Read the model definition and answer for the solid it produces. Units are mm, in the model's axes. A direction names the side the tool comes from. Round coordinates to 2 decimals unless told otherwise and drop trailing zeros. Order: outer loops, then holes, each group sorted by start corner. A loop starts at its lowest first (then second) coordinate and runs counter-clockwise, first axis right, second up. Notation, with made-up numbers: (-35.75, 66) - (1.25, 66) arc R18 ccw to (1.25, 71) - close; hole circle Ø3 at (89, 79.25). An arc over 180 degrees is marked (long way). Answer as a JSON object with one key per item and string values. Group by question number.
Q1. Given pin 1 Ø1.5 at (x, z) = (-5, 4) entering from -Y; pin 2 Ø0.6 at (y, z) = (-1.5, 0.5) entering from -X; pin 3 Ø3 at (x, y) = (-7, -2.5) entering from +Z; pin 4 Ø2.5 at (x, z) = (11, 3.5) entering from -Y, each flat-ended and moving along its own axis, determine where each tip first touches the part or whether it passes through.
Q2. Consider line 1 (Z direction, x = -11, y = -11.2); line 2 (X direction, y = 5, z = 0.75); line 3 (Z direction, x = -8.75, y = 4.5). Determine where each line is inside the solid, lowest interval first.
Q3. A cutting plane is placed at A-A on z = 1.5. Determine the outline of the cut face in (x, y).
Q4. A cutting plane is placed at C-C on x = -10.5. Determine the outline of the cut face in (y, z), and give its area (3 significant figures).
Q5. A cutting plane is placed at D-D on z = 3.5. Count the separate pieces of the cut face and the enclosed holes in it, and give its area (3 significant figures).
Q6. The mould has two halves that part along Y. Classify faces 5 (the flat face through (-6, 10, 4)), 6 (the flat face through (9, -10, 4)), 7 (the cylindrical face through (9.5, -7.46, 3.57)): pulls with the +Y half, pulls with the -Y half, needs draft (parallel to the pull), parting line crosses it, or undercut.
Q7. A tool of negligible diameter and unlimited length cuts with its end or side. For faces 1 (the flat face through (10.5, 7.5, 1)), 2 (the flat face through (-7, -15, 4)), 3 (the cylindrical face through (7.056, -10.245, 3.465)), 4 (the flat face through (-10.5, 12.5, 1)), from which of +Z, -Z, +X, -X, +Y, -Y can it reach the whole face along a straight path? Write none if from no direction.
Q8. A cutting plane is placed at B-B on y = 12. Determine the outline of the cut face in (x, z), and give its area (3 significant figures).
```python
from build123d import *

# Parameters (mm, degrees)
F0_W          = 20
F0_H          = 1
F1_DEPTH      = 20
F1_DEPTH_BACK = 20
F3_DEPTH      = 40
F5_DEPTH      = 5
F7_R          = 1.5
F8_DEPTH      = 20.001
F8_DEPTH_BACK = 20.001
F9_R          = 5


# Not quite as in the source:
# - a pattern or mirror of a feature is missing from the dataset's text; its kind, count and spacing are read off the source's solid


with BuildPart() as f1:
    # F0 (on Front) → F1 (new body, two sides)
    with BuildSketch(Plane.XZ) as f1_sk:
        with Locations((0, -0.5)):
            Rectangle(F0_W, F0_H)
    extrude(amount=F1_DEPTH)
    extrude(f1_sk.sketch, amount=-F1_DEPTH_BACK)

    # F2 (on face) → F3 (join, through all)
    with BuildSketch(Plane(origin=(0, 20, 0), x_dir=(-1, 0, 0), z_dir=(0, 1, 0))):
        with BuildLine():
            Line((10, 1), (11, 1))
            ThreePointArc((11, 1), (13.5, 3.5), (11, 6))
            Line((11, 6), (0, 6))
            Line((0, 6), (-11, 6))
            ThreePointArc((-11, 6), (-13.5, 3.5), (-11, 1))
            Line((-11, 1), (-10, 1))
            Line((-10, 1), (-10, 0))
            Line((-10, 0), (0, 0))
            Line((0, 0), (10, 0))
            Line((10, 0), (10, 1))
        make_face()
    extrude(amount=-F3_DEPTH)

    # F4 (on face) → F5 (cut, through all)
    with BuildSketch(Plane.XY.offset(6)):
        Polygon((0, -15), (-13.5, -15), (-13.5, -20), (13.5, -20), (13.5, -10), (7, -10), align=None)
        Polygon((-13.5, 0), (-13.5, -10), (0, -10), (7, -5), (13.5, -5), (13.5, 0), align=None)
    f5 = extrude(amount=-F5_DEPTH, mode=Mode.SUBTRACT)

    # F5_copies: F5 across plane
    add(f5.mirror(Plane.ZX), mode=Mode.SUBTRACT)

    # F7 (on offset) → F8 (cut, two sides)
    with BuildSketch(Plane.XZ) as f8_sk:
        with Locations((11, 3.5)):
            Circle(F7_R)
        with Locations((-11, 3.5)):
            Circle(F7_R)
    extrude(amount=-F8_DEPTH, mode=Mode.SUBTRACT)
    extrude(f8_sk.sketch, amount=F8_DEPTH_BACK, mode=Mode.SUBTRACT)

    # F9
    f9_edges = [f1.edges().sort_by_distance(p)[0] for p in [
        (0, -15, 3.5),
        (0, -10, 3.5),
        (7, -5, 3.5),
        (7, -10, 3.5),
        (7, 10, 3.5),
        (0, 15, 3.5),
        (0, 10, 3.5),
        (7, 5, 3.5),
    ]]
    fillet(f9_edges, radius=F9_R)


solid = f1.part
```
Result set:
{
 "1": {"pin 1": "stops at y = -15", "pin 2": "stops at x = -10", "pin 3": "stops at z = 1", "pin 4": "passes through"},
 "2": {"line 1": "z = 1 to 2, 5 to 6", "line 2": "x = -10 to 10", "line 3": "z = -1 to 1"},
 "3": {"outline": "(-12.5, -15) - (-1.6, -15) arc R5 ccw to (1.3, -14.07) - (5.7, -10.93) arc R5 cw to (8.6, -10) - (12.5, -10) - (12.5, -5) - (8.6, -5) arc R5 ccw to (5.7, -5.93) - (1.3, -9.07) arc R5 cw to (-1.6, -10) - (-12.5, -10) - close; (-12.5, 10) - (-1.6, 10) arc R5 cw to (1.3, 9.07) - (5.7, 5.93) arc R5 ccw to (8.6, 5) - (12.5, 5) - (12.5, 10) - (8.6, 10) arc R5 cw to (5.7, 10.93) - (1.3, 14.07) arc R5 ccw to (-1.6, 15) - (-12.5, 15) - close"},
 "4": {"outline": "(-15, 1) - (-10, 1) - (-10, 2.09) - (-15, 2.09) - close; (-15, 4.91) - (-10, 4.91) - (-10, 6) - (-15, 6) - close; (10, 1) - (15, 1) - (15, 2.09) - (10, 2.09) - close; (10, 4.91) - (15, 4.91) - (15, 6) - (10, 6) - close", "area": "21.7 mm²"},
 "5": {"separate pieces": "6", "enclosed holes": "0", "area": "210 mm²"},
 "6": {"face 5": "undercut", "face 6": "pulls with the -Y half", "face 7": "needs draft"},
 "7": {"face 1": "-Z, +X, +Y, -Y", "face 2": "+Z, +X, -X, -Y", "face 3": "+Z, +X, -Y", "face 4": "-Z, -X, +Y, -Y"},
 "8": {"outline": "(-11, 1) - (-10, 1) - (-10, -1) - (10, -1) - (10, 1) - (4.2, 1) - (4.2, 6) - (-11, 6) arc R2.5 ccw to start; hole circle Ø3 at (-11, 3.5)", "area": "119 mm²"}
}
